Autodesk Inventor part; units mm, degrees
ref_plane "YZ Plane" through (0, 0, 0) normal (1, 0, 0) x (0, 1, 0)
ref_plane "XZ Plane" through (0, 0, 0) normal (0, 1, 0) x (-1, 0, 0)
ref_plane "XY Plane" through (0, 0, 0) normal (0, 0, 1) x (1, 0, 0)
sketch "スケッチ1" plane through (0, 0, 0) normal (0, 0, 1) x (1, 0, 0)
  line L0 (-12, 12) -> (12, 12)
  line L1 (12, 12) -> (12, -12)
  line L2 (12, -12) -> (-12, -12)
  line L3 (-12, -12) -> (-12, 12)
  line L4 (-12, 12) -> (12, -12) construction
  line L5 (12, 12) -> (-12, -12) construction
  point P0 (0, 0)
  dimension "d0" = 24
  dimension "d1" = 24
extrude "押し出し1" add sketch "スケッチ1" along normal blind 14
fillet "フィレット1" radius 4 4 edges at (-12, 12, 7) (12, 12, 7) (12, -12, 7) (-12, -12, 7)
sketch "スケッチ2" plane through (0, 0, 14) normal (0, 0, 1) x (1, 0, 0)
  arc A0 (-12, -8) -> (-8, -12) centre (-8, -8) ccw
  line L0 (-8, -12) -> (8, -12)
  arc A1 (8, -12) -> (12, -8) centre (8, -8) ccw
  line L1 (12, -8) -> (12, 8)
  arc A2 (12, 8) -> (8, 12) centre (8, 8) ccw
  line L2 (8, 12) -> (-8, 12)
  arc A3 (-8, 12) -> (-12, 8) centre (-8, 8) ccw
  line L3 (-12, 8) -> (-12, -8)
  line L4 (-8, 10.5) -> (8, 10.5)
  arc A4 (10.5, 8) -> (8, 10.5) centre (8, 8) ccw
  line L5 (10.5, 8) -> (10.5, -8)
  arc A5 (8, -10.5) -> (10.5, -8) centre (8, -8) ccw
  line L6 (8, -10.5) -> (-8, -10.5)
  arc A6 (-10.5, -8) -> (-8, -10.5) centre (-8, -8) ccw
  line L7 (-10.5, -8) -> (-10.5, 8)
  arc A7 (-8, 10.5) -> (-10.5, 8) centre (-8, 8) ccw
  point P0 (0, 0)
  dimension "d5" = 1.5
extrude "押し出し2" cut sketch "スケッチ2" against normal blind 1 contours L4 A4 L5 A5 L6 A6 L7 A7
properties part number "M5Atom"
Geometry check sheet. Reference: the model listing, model coordinates, mm. A direction names the side the tool comes from. Give positions to 0.01 mm unless a question says otherwise; leave off trailing zeros. Write each loop counter-clockwise with the first axis right and the second up, starting at its lowest first coordinate (ties: lowest second). Pieces come first, ordered by that corner, then holes.
1) Material ranges on L1, parallel to Z at x = 2.25, y = 4; L2, parallel to Y at x = 9, z = 13.25; L3, parallel to X at y = 9.5, z = 11, recorded low to high.
2) Section check B-B, the plane z = 3.5. Record the boundary of the cut face in (x, y), and give its area (3 significant figures).
3) Gauge pin test, flat ends, axial feed: pin 1 (1 mm diameter, centred on x = 9, z = 8, fed in from +Y); pin 2 (5 mm diameter, centred on y = -8.5, z = 11.5, fed in from -X); pin 3 (6.5 mm diameter, centred on x = 4, y = -4, fed in from +Z). Record the tip position at first contact, or that the pin passes through.
4) Section check A-A, the plane y = 7.5. Record the boundary of the cut face in (x, z).
5) Access from +Z, -Z, +X, -X, +Y, -Y to the whole of each face (thin tool, end or side, straight path). Record for faces 1 (the flat face through (0.1, -10.5, 13.5)), 2 (the flat face through (12, 0, 7)).
Computed:
1. L1: z = 0 to 13
1. L2: y = -11.87 to -10.29, 10.29 to 11.87
1. L3: x = -11.71 to 11.71
2. outline: (-12, -8) arc R4 ccw to (-8, -12) - (8, -12) arc R4 ccw to (12, -8) - (12, 8) arc R4 ccw to (8, 12) - (-8, 12) arc R4 ccw to (-12, 8) - close
2. area: 562 mm2
3. pin 1: stops at y = 11.97
3. pin 2: stops at x = -12
3. pin 3: stops at z = 13
4. outline: (-12, 0) - (12, 0) - (12, 14) - (10.5, 14) - (10.5, 13) - (-10.5, 13) - (-10.5, 14) - (-12, 14) - close
5. face 1: +Z
5. face 2: +Z, -Z, +X, +Y, -Y
